from build123d import *

# Parameters (mm, degrees)
SKETCH_1_R           = 1.7
EXTRUDE_6_DEPTH      = 4
EXTRUDE_7_DEPTH      = 100
SKETCH_10_W          = 140
SKETCH_10_H          = 96
CUT_EXTRUDE_20_DEPTH = 115
CUT_EXTRUDE_START    = -148
SKETCH_16_R          = 1.5
SKETCH_16_R_2        = 4
CUT_EXTRUDE_22_DEPTH = 148
SKETCH_21_W          = 110
SKETCH_21_H          = 80
CUT_EXTRUDE_28_DEPTH = 50
SKETCH_23_R          = 5
CUT_EXTRUDE_29_DEPTH = 148
SKETCH_31_W          = 143.9
SKETCH_31_H          = 99.9
SKETCH_31_W_2        = 140
SKETCH_31_H_2        = 96
EXTRUDE_9_DEPTH      = 10
CUT_EXTRUDE_START_2  = -99.9
SKETCH_32_R          = 2
CUT_EXTRUDE_32_DEPTH = 99.9
CUT_EXTRUDE_START_3  = -143.9
SKETCH_33_R          = 2
CUT_EXTRUDE_33_DEPTH = 143.9


with BuildPart() as part:
    # 草图1 → 凸台-拉伸6 (new body)
    with BuildSketch(Plane(origin=(0, 0, 0), x_dir=(1, 0, 0), z_dir=(0, 1, 0))):
        with BuildLine():
            Line((-74, 0), (-74, -115))
            ThreePointArc((-74, -115), (-71.363961031, -121.363961031), (-65, -124))
            Line((-65, -124), (65, -124))
            ThreePointArc((65, -124), (71.363961031, -121.363961031), (74, -115))
            Line((74, -115), (74, 0))
            Line((74, 0), (-74, 0))
        make_face()
        with Locations(Location((-62, -108, 0), (0, 0, 270))):
            Circle(SKETCH_1_R, mode=Mode.SUBTRACT)
        with Locations(Location((-48, -108, 0), (0, 0, 270))):
            Circle(SKETCH_1_R, mode=Mode.SUBTRACT)
        with Locations(Location((48, -108, 0), (0, 0, 270))):
            Circle(SKETCH_1_R, mode=Mode.SUBTRACT)
        with Locations(Location((62, -108, 0), (0, 0, 270))):
            Circle(SKETCH_1_R, mode=Mode.SUBTRACT)
        with Locations(Location((-62, -92, 0), (0, 0, 270))):
            Circle(SKETCH_1_R, mode=Mode.SUBTRACT)
        with Locations(Location((-48, -92, 0), (0, 0, 270))):
            Circle(SKETCH_1_R, mode=Mode.SUBTRACT)
        with BuildLine():
            ThreePointArc((-25, -90), (-23.535533906, -86.464466094), (-20, -85))
            Line((-20, -85), (20, -85))
            ThreePointArc((20, -85), (23.535533906, -86.464466094), (25, -90))
            Line((25, -90), (25, -107.989151936))
            ThreePointArc((25, -107.989151936), (23.535533906, -111.524685842), (20, -112.989151936))
            Line((20, -112.989151936), (-20, -112.989151936))
            ThreePointArc((-20, -112.989151936), (-23.535533906, -111.524685842), (-25, -107.989151936))
            Line((-25, -107.989151936), (-25, -90))
        make_face(mode=Mode.SUBTRACT)
        with Locations(Location((48, -92, 0), (0, 0, 270))):
            Circle(SKETCH_1_R, mode=Mode.SUBTRACT)
        with Locations(Location((62, -92, 0), (0, 0, 270))):
            Circle(SKETCH_1_R, mode=Mode.SUBTRACT)
    extrude(amount=EXTRUDE_6_DEPTH)

    # 草图9 → 凸台-拉伸7 (add)
    with BuildSketch(Plane(origin=(0, 4, 0), x_dir=(1, 0, 0), z_dir=(0, 1, 0))):
        with BuildLine():
            Line((-74, 0), (74, 0))
            Line((74, 0), (74, -115.166586314))
            ThreePointArc((74, -115.166586314), (71.363961031, -121.530547345), (65, -124.166586314))
            Line((65, -124.166586314), (-65, -124.166586314))
            ThreePointArc((-65, -124.166586314), (-71.363961031, -121.530547345), (-74, -115.166586314))
            Line((-74, -115.166586314), (-74, 0))
        make_face()
    extrude(amount=EXTRUDE_7_DEPTH)

    # 草图10 → 切除-拉伸20 (cut)
    with BuildSketch(Plane(origin=(0, 0, 0), x_dir=(-1, 0, 0), z_dir=(0, 0, -1))):
        with Locations((0, 52)):
            Rectangle(SKETCH_10_W, SKETCH_10_H)
    extrude(amount=-CUT_EXTRUDE_20_DEPTH, mode=Mode.SUBTRACT)

    # 草图16 → 切除-拉伸22 (cut)
    with BuildSketch(Plane.ZY.offset(74).offset(CUT_EXTRUDE_START)):
        with Locations(Location((100, 16.25, 0), (0, 0, 180))):
            Circle(SKETCH_16_R)
        with Locations(Location((108.5, 24.75, 0), (0, 0, 180))):
            Circle(SKETCH_16_R)
        with Locations(Location((100, 24.75, 0), (0, 0, 180))):
            Circle(SKETCH_16_R_2)
        with Locations(Location((91.5, 24.75, 0), (0, 0, 180))):
            Circle(SKETCH_16_R)
        with Locations(Location((100, 33.25, 0), (0, 0, 180))):
            Circle(SKETCH_16_R)
    extrude(amount=CUT_EXTRUDE_22_DEPTH, mode=Mode.SUBTRACT)

    # 草图21 → 切除-拉伸28 (cut)
    with BuildSketch(Plane.XY.offset(124.166586314)):
        with Locations((0, 54)):
            Rectangle(SKETCH_21_W, SKETCH_21_H)
    extrude(amount=-CUT_EXTRUDE_28_DEPTH, mode=Mode.SUBTRACT)

    # 草图23 → 切除-拉伸29 (cut)
    with BuildSketch(Plane.ZY.offset(74).offset(CUT_EXTRUDE_START)):
        with Locations((100, 24.75)):
            Circle(SKETCH_23_R)
    extrude(amount=CUT_EXTRUDE_29_DEPTH, mode=Mode.SUBTRACT)

    # 草图31 → 凸台-拉伸9 (add)
    with BuildSketch(Plane(origin=(0, 0, 0), x_dir=(-1, 0, 0), z_dir=(0, 0, -1))):
        with Locations((0, 52)):
            Rectangle(SKETCH_31_W, SKETCH_31_H)
        with Locations((0, 52)):
            Rectangle(SKETCH_31_W_2, SKETCH_31_H_2, mode=Mode.SUBTRACT)
    extrude(amount=EXTRUDE_9_DEPTH)

    # 草图32 → 切除-拉伸32 (cut)
    with BuildSketch(Plane(origin=(0, 101.95, 0), x_dir=(1, 0, 0), z_dir=(0, 1, 0)).offset(CUT_EXTRUDE_START_2)):
        with Locations(Location((0, 5, 0), (0, 0, 180))):
            Circle(SKETCH_32_R)
        with Locations(Location((20, 5, 0), (0, 0, 180))):
            Circle(SKETCH_32_R)
        with Locations(Location((40, 5, 0), (0, 0, 180))):
            Circle(SKETCH_32_R)
        with Locations(Location((60, 5, 0), (0, 0, 180))):
            Circle(SKETCH_32_R)
        with Locations(Location((-60, 5, 0), (0, 0, 180))):
            Circle(SKETCH_32_R)
        with Locations(Location((-20, 5, 0), (0, 0, 180))):
            Circle(SKETCH_32_R)
        with Locations(Location((-40, 5, 0), (0, 0, 180))):
            Circle(SKETCH_32_R)
    extrude(amount=CUT_EXTRUDE_32_DEPTH, mode=Mode.SUBTRACT)

    # 草图33 → 切除-拉伸33 (cut)
    with BuildSketch(Plane.ZY.offset(71.95).offset(CUT_EXTRUDE_START_3)):
        with Locations(Location((-5, 52, 0), (0, 0, 90))):
            Circle(SKETCH_33_R)
        with Locations(Location((-5, 72, 0), (0, 0, 90))):
            Circle(SKETCH_33_R)
        with Locations(Location((-5, 92, 0), (0, 0, 90))):
            Circle(SKETCH_33_R)
        with Locations(Location((-5, 12, 0), (0, 0, 90))):
            Circle(SKETCH_33_R)
        with Locations(Location((-5, 32, 0), (0, 0, 90))):
            Circle(SKETCH_33_R)
    extrude(amount=CUT_EXTRUDE_33_DEPTH, mode=Mode.SUBTRACT)


solid = part.part
CAD build for the part. Positions are in the model's coordinates, mm. A direction names the side the tool comes from. Give positions to 0.01 mm unless a question says otherwise; leave off trailing zeros. Order: outer loops, then holes, each group sorted by start corner. A loop starts at its lowest first (then second) coordinate and runs counter-clockwise, first axis right, second up. Notation, with made-up numbers: (1, 39.25) -> (45, 39.25) arc R14 cw to (45, 51.25) -> close; hole circle Ø2 at (58.25, 35). An arc over 180 degrees is marked (long way). Return JSON: item names as keys, results as strings.
Q1. Saw through at A-A (z = 43). Write the cut outline in (x, y).
Working result:
{"outline": "(-74, 0) -> (74, 0) -> (74, 104) -> (-74, 104) -> close; hole (-70, 4) -> (70, 4) -> (70, 100) -> (-70, 100) -> close"}
Q2. Flat gauge pins, fed straight in: pin 1 (6.5 mm diameter, centred on x = -20, z = -5, fed in from +Y); pin 2 (4.5 mm diameter, centred on y = 72, z = -5, fed in from +X); pin 3 (2 mm diameter, centred on x = -62, z = 108, fed in from -Y). Where does each tip first touch, or does it go through?
Working result:
{"pin 1": "y = 101.95", "pin 2": "x = 71.95", "pin 3": "y = 100"}
Q3. Drill centre lines: line 1 (Y direction, x = -70.35, z = -5); line 2 (Y direction, x = 30.5, z = 37); line 3 (X direction, y = 63, z = 45). Where is each one in solid material? Low to high.
Working result:
{"line 1": "2.05 to 10, 14 to 30, 34 to 50, 54 to 70, 74 to 90, 94 to 101.95", "line 2": "0 to 4, 100 to 104", "line 3": "-74 to -70, 70 to 74"}
Q4. Mould opens along Z. For faces 1 (the face through (-1, 94, 120)), 2 (the face through (21.6, 3, -6.2)), 3 (the face through (70.989, 33.908, -5.601)), 4 (the face through (-1, 2, 124)) say: pulls with the +Z half, pulls with the -Z half, needs draft (parallel to the pull), parting line crosses it, or undercut.
Working result:
{"face 1": "needs draft", "face 2": "undercut", "face 3": "undercut", "face 4": "pulls with the +Z half"}
Q5. Which spindle directions (+Z, -Z, +X, -X, +Y, -Y) get a long thin tool onto all of the face, cutting with end or side? Do faces 5 (the face through (1, 4, 53)), 6 (the face through (71.294, 1.972, 121.434)), 7 (the face through (-71.95, 51, -3)), 8 (the face through (48.07, 1.97, 106.3)). Say none if no direction does.
Working result:
{"face 5": "-Z", "face 6": "+Z, +X, -Y", "face 7": "-Z, -X, +Y, -Y", "face 8": "-Y"}
Q6. Saw through at B-B (y = 72). Write the cut outline in (x, z), then the cut area to 3 significant figures.
Working result:
{"outline": "(-74, 0) -> (-71.95, 0) -> (-71.95, -3) -> (-70, -3) -> (-70, 115) -> (-55, 115) -> (-55, 124.17) -> (-65, 124.17) arc R9 ccw to (-74, 115.17) -> close; (-71.95, -10) -> (-70, -10) -> (-70, -7) -> (-71.95, -7) -> close; (55, 115) -> (70, 115) -> (70, -3) -> (71.95, -3) -> (71.95, 0) -> (74, 0) -> (74, 115.17) arc R9 ccw to (65, 124.17) -> (55, 124.17) -> close; (70, -10) -> (71.95, -10) -> (71.95, -7) -> (70, -7) -> close", "area": "1,260 mm²"}
Q7. Saw through at C-C (x = 53). Write the cut outline in (y, z), then the cut area to 3 significant figures.
Working result:
{"outline": "(0, 0) -> (2.05, 0) -> (2.05, -10) -> (4, -10) -> (4, 115) -> (14, 115) -> (14, 124.17) -> (4, 124.17) -> (4, 124) -> (0, 124) -> close; (94, 115) -> (100, 115) -> (100, -10) -> (101.95, -10) -> (101.95, 0) -> (104, 0) -> (104, 124.17) -> (94, 124.17) -> close", "area": "1,180 mm²"}
